The model under review builds one solid part; all positions refer to its coordinate system, in mm. A direction names the side the tool comes from. Round coordinates to 2 decimals unless told otherwise and drop trailing zeros. Write each loop counter-clockwise with the first axis right and the second up, starting at its lowest first coordinate (ties: lowest second). Pieces come first, ordered by that corner, then holes. Notation, with made-up numbers: (27, -36.5) - (34, -36.5) arc R14 cw to (34, -13.5) - close; hole circle Ø6 at (-13.5, 78). An arc over 180 degrees is marked (long way). Return JSON: item names as keys, results as strings.
from build123d import *

# Parameters (mm, degrees)
SALIENTE_EXTRUIR1_DEPTH = 27
CROQUIS3_R              = 4
CROQUIS3_R_2            = 2
SALIENTE_EXTRUIR2_DEPTH = 2
CROQUIS6_R              = 2
CORTAR_EXTRUIR2_DEPTH   = 10
SALIENTE_EXTRUIR4_START = 2
CROQUIS9_R              = 4
CROQUIS9_R_2            = 2
SALIENTE_EXTRUIR4_DEPTH = 2
CORTAR_EXTRUIR3_START   = -10
CROQUIS10_R             = 2
CORTAR_EXTRUIR3_DEPTH   = 10
CROQUIS11_R             = 9.5
SALIENTE_EXTRUIR5_DEPTH = 4.5
SALIENTE_EXTRUIR6_START = 4.5
CROQUIS12_R             = 9.5
SALIENTE_EXTRUIR6_DEPTH = 4.5
CROQUIS13_R             = 4
SALIENTE_EXTRUIR7_DEPTH = 15
CORTAR_EXTRUIR6_START   = -13
CORTAR_EXTRUIR6_DEPTH   = 13
SALIENTE_EXTRUIR8_START = 15
CROQUIS16_R             = 4
SALIENTE_EXTRUIR8_DEPTH = 15
CORTAR_EXTRUIR7_DEPTH   = 13
CROQUIS18_R             = 4
CORTAR_EXTRUIR8_DEPTH   = 20


with BuildPart() as part:
    # Croquis2 → Saliente-Extruir1 (new body)
    with BuildSketch(Plane(origin=(0, 0, 0), x_dir=(1, 0, 0), z_dir=(0, 1, 0))):
        with BuildLine():
            Line((-26.320513929, 20.055), (26.15, 20.055))
            ThreePointArc((26.15, 20.055), (28.26352098, 19.143001272), (29.05, 16.97963275))
            Line((29.05, 16.97963275), (29.05, -16.97963275))
            ThreePointArc((29.05, -16.97963275), (28.26352098, -19.143001272), (26.15, -20.055))
            Line((26.15, -20.055), (-26.320513929, -20.055))
            ThreePointArc((-26.320513929, -20.055), (-28.26710835, -19.146484969), (-29.06, -17.15))
            Line((-29.06, -17.15), (-29.06, 17.15))
            ThreePointArc((-29.06, 17.15), (-28.26710835, 19.146484969), (-26.320513929, 20.055))
        make_face()
    extrude(amount=SALIENTE_EXTRUIR1_DEPTH)

    # Croquis3 → Saliente-Extruir2 (add)
    with BuildSketch(Plane(origin=(0, 27, 0), x_dir=(1, 0, 0), z_dir=(0, 1, 0))):
        with BuildLine():
            Line((22.293849377, -10.723072318), (19.016921695, -8.42922294))
            ThreePointArc((19.016921695, -8.42922294), (13.446144636, -9.412301245), (14.42922294, -14.983078305))
            Line((14.42922294, -14.983078305), (17.706150623, -17.276927682))
            ThreePointArc((17.706150623, -17.276927682), (23.276927682, -16.293849377), (22.293849377, -10.723072318))
        make_face()
        with Locations(Location((-20, 14, 0), (0, 0, 270))):
            Circle(CROQUIS3_R)
        with Locations(Location((20, 14, 0), (0, 0, 270))):
            Circle(CROQUIS3_R)
        with Locations(Location((-20, -14, 0), (0, 0, 270))):
            Circle(CROQUIS3_R)
        with Locations(Location((8, 4, 0), (0, 0, 270))):
            Circle(CROQUIS3_R_2)
        with Locations(Location((8, -4, 0), (0, 0, 270))):
            Circle(CROQUIS3_R_2)
    extrude(amount=SALIENTE_EXTRUIR2_DEPTH)

    # Croquis6 → Cortar-Extruir2 (cut)
    with BuildSketch(Plane(origin=(0, 29, 0), x_dir=(1, 0, 0), z_dir=(0, 1, 0))):
        with Locations(Location((-20, 14, 0), (0, 0, 270))):
            Circle(CROQUIS6_R)
        with Locations(Location((20, 14, 0), (0, 0, 270))):
            Circle(CROQUIS6_R)
        with Locations(Location((20, -14, 0), (0, 0, 270))):
            Circle(CROQUIS6_R)
        with Locations(Location((-20, -14, 0), (0, 0, 270))):
            Circle(CROQUIS6_R)
    extrude(amount=-CORTAR_EXTRUIR2_DEPTH, mode=Mode.SUBTRACT)

    # Croquis9 → Saliente-Extruir4 (add)
    with BuildSketch(Plane.XZ.offset(SALIENTE_EXTRUIR4_START)):
        with Locations(Location((-20, 14, 0), (0, 0, 90))):
            Circle(CROQUIS9_R)
        with Locations(Location((-20, -14, 0), (0, 0, 90))):
            Circle(CROQUIS9_R)
        with Locations(Location((8, 4, 0), (0, 0, 90))):
            Circle(CROQUIS9_R_2)
        with Locations(Location((8, -4, 0), (0, 0, 90))):
            Circle(CROQUIS9_R_2)
        with Locations(Location((20, -14, 0), (0, 0, 90))):
            Circle(CROQUIS9_R)
        with BuildLine():
            Line((14.255148366, 14.861221242), (17.535309468, 17.150444505))
            ThreePointArc((17.535309468, 17.150444505), (23.214821143, 16.380110295), (22.293849377, 10.723072318))
            Line((22.293849377, 10.723072318), (18.838221007, 8.304132458))
            ThreePointArc((18.838221007, 8.304132458), (13.265826422, 9.28952325), (14.255148366, 14.861221242))
        make_face()
    extrude(amount=-SALIENTE_EXTRUIR4_DEPTH)

    # Croquis10 → Cortar-Extruir3 (cut)
    with BuildSketch(Plane.XZ.offset(2).offset(CORTAR_EXTRUIR3_START)):
        with Locations(Location((20, -14, 0), (0, 0, 90))):
            Circle(CROQUIS10_R)
        with Locations(Location((20, 14, 0), (0, 0, 90))):
            Circle(CROQUIS10_R)
        with Locations(Location((-20, 14, 0), (0, 0, 90))):
            Circle(CROQUIS10_R)
        with Locations(Location((-20, -14, 0), (0, 0, 90))):
            Circle(CROQUIS10_R)
    extrude(amount=CORTAR_EXTRUIR3_DEPTH, mode=Mode.SUBTRACT)

    # Croquis11 → Saliente-Extruir5 (add)
    with BuildSketch(Plane(origin=(0, 27, 0), x_dir=(1, 0, 0), z_dir=(0, 1, 0))):
        with Locations(Location((-8.85, 0, 0), (0, 0, 270))):
            Circle(CROQUIS11_R)
    extrude(amount=SALIENTE_EXTRUIR5_DEPTH)

    # Croquis12 → Saliente-Extruir6 (add)
    with BuildSketch(Plane.XZ.offset(SALIENTE_EXTRUIR6_START)):
        with Locations(Location((-8.85, 0, 0), (0, 0, 90))):
            Circle(CROQUIS12_R)
    extrude(amount=-SALIENTE_EXTRUIR6_DEPTH)

    # Croquis13 → Saliente-Extruir7 (add)
    with BuildSketch(Plane(origin=(0, 31.5, 0), x_dir=(1, 0, 0), z_dir=(0, 1, 0))):
        with Locations(Location((-8.85, 0, 0), (0, 0, 270))):
            Circle(CROQUIS13_R)
    extrude(amount=SALIENTE_EXTRUIR7_DEPTH)

    # Croquis15 → Cortar-Extruir6 (cut)
    with BuildSketch(Plane(origin=(0, 46.5, 0), x_dir=(1, 0, 0), z_dir=(0, 1, 0)).offset(CORTAR_EXTRUIR6_START)):
        with BuildLine():
            Line((-5.85, 2.645751311), (-5.85, -2.645751311))
            ThreePointArc((-5.85, -2.645751311), (-4.85, 0), (-5.85, 2.645751311))
        make_face()
    extrude(amount=CORTAR_EXTRUIR6_DEPTH, mode=Mode.SUBTRACT)

    # Croquis16 → Saliente-Extruir8 (add)
    with BuildSketch(Plane.XZ.offset(4.5).offset(SALIENTE_EXTRUIR8_START)):
        with Locations(Location((-8.85, 0, 0), (0, 0, 318.590377891))):
            Circle(CROQUIS16_R)
    extrude(amount=-SALIENTE_EXTRUIR8_DEPTH)

    # Croquis17 → Cortar-Extruir7 (cut)
    with BuildSketch(Plane.XZ.offset(19.5)):
        with BuildLine():
            Line((-5.85, 2.645751311), (-5.85, -2.645751311))
            ThreePointArc((-5.85, -2.645751311), (-4.85, 0), (-5.85, 2.645751311))
        make_face()
    extrude(amount=-CORTAR_EXTRUIR7_DEPTH, mode=Mode.SUBTRACT)

    # Croquis18 → Cortar-Extruir8 (cut)
    with BuildSketch(Plane(origin=(29.05, 0, 0), x_dir=(0, 0, -1), z_dir=(1, 0, 0))):
        with Locations((0, 11.5)):
            Circle(CROQUIS18_R)
    extrude(amount=-CORTAR_EXTRUIR8_DEPTH, mode=Mode.SUBTRACT)


solid = part.part
(1) For faces 5 (the flat face through (8, 29, 4)), 6 (the flat face through (18, -2, 13)), 7 (the cylindrical face through (-22.7, -1.01, -16.95)), 8 (the flat face through (9.05, 12, 0)), 9 (the cylindrical face through (-17.3, 27.99, -16.95)), list the 3-axis set-ups (+Z, -Z, +X, -X, +Y, -Y) from which the entire face can be reached by the end or side of a thin tool; tool diameter is ignored.
Filled in:
{"face 5": "+Z, -Z, +X, +Y", "face 6": "+Z, -Z, +X, -Y", "face 7": "-Y", "face 8": "+X", "face 9": "+Y"}
(2) Add section C-C (y = 11.5). Write out the cut boundary in (x, z) (3 decimals), plus the area to 3 significant figures.
Filled in:
{"outline": "(-29.06, -17.15) arc R2.91 ccw to (-26.321, -20.055) - (26.15, -20.055) arc R2.905 ccw to (29.05, -16.98) - (29.05, -4) - (9.05, -4) - (9.05, 4) - (29.05, 4) - (29.05, 16.98) arc R2.905 ccw to (26.15, 20.055) - (-26.321, 20.055) arc R2.91 ccw to (-29.06, 17.15) - close", "area": "2,160 mm2"}
(3) Mouldability with a two-part tool opening along Y and no side actions: class faces 1 (the cylindrical face through (19.19, 15.466, 0.521)), 2 (the flat face through (8, -2, -4)), 3 (the flat face through (-9, 46.5, 0)), 4 (the flat face through (29.05, 16, 0)) as released by +Y, released by -Y, zero draft, split by the parting line, or undercut.
Filled in:
{"face 1": "undercut", "face 2": "released by -Y", "face 3": "released by +Y", "face 4": "zero draft"}
(4) Add section D-D (z = 5). Write out the cut boundary in (x, y), plus the area to 3 significant figures.
Filled in:
{"outline": "(-29.06, 0) - (-16.93, 0) - (-16.93, -4.5) - (-0.77, -4.5) - (-0.77, 0) - (6.27, 0) - (6.27, -2) - (9.73, -2) - (9.73, 0) - (29.05, 0) - (29.05, 27) - (9.73, 27) - (9.73, 29) - (6.27, 29) - (6.27, 27) - (-0.77, 27) - (-0.77, 31.5) - (-16.93, 31.5) - (-16.93, 27) - (-29.06, 27) - close", "area": "1,730 mm2"}
(5) Add section B-B (z = 0). Write out the cut boundary in (x, y), plus the area to 3 significant figures.
Filled in:
{"outline": "(-29.06, 0) - (-18.35, 0) - (-18.35, -4.5) - (-12.85, -4.5) - (-12.85, -19.5) - (-5.85, -19.5) - (-5.85, -6.5) - (-4.85, -6.5) - (-4.85, -4.5) - (0.65, -4.5) - (0.65, 0) - (29.05, 0) - (29.05, 7.5) - (9.05, 7.5) - (9.05, 15.5) - (29.05, 15.5) - (29.05, 27) - (0.65, 27) - (0.65, 31.5) - (-4.85, 31.5) - (-4.85, 33.5) - (-5.85, 33.5) - (-5.85, 46.5) - (-12.85, 46.5) - (-12.85, 31.5) - (-18.35, 31.5) - (-18.35, 27) - (-29.06, 27) - close", "area": "1,790 mm2"}
(6) Wall thickness on line 1 (Z direction, x = 20, y = 2.5) (3 decimals); line 2 (X direction, y = 20, z = -14); line 3 (Z direction, x = 19.5, y = 4) (1 decimal): over which ranges is each line inside the solid? List them lowest first.
Filled in:
{"line 1": "z = -20.055 to -16, -12 to 12, 16 to 20.055", "line 2": "x = -29.06 to -22, -18 to 18, 22 to 29.05", "line 3": "z = -20.1 to -15.9, -12.1 to 12.1, 15.9 to 20.1"}
(7) Clearance check with flat-ended pins moving along their axes: pin 1 Ø9 at (x, z) = (-19.5, -14) entering from +Y; pin 2 Ø2 at (x, z) = (20, -14.5) entering from -Y; pin 3 Ø1.5 at (x, z) = (-19.5, -8) entering from -Y. State where each tip first meets the part, or that it passes through.
Filled in:
{"pin 1": "stops at y = 29", "pin 2": "stops at y = 8", "pin 3": "stops at y = 0"}
(8) Add section A-A (x = 25). Write out the cut boundary in (y, z) (3 decimals).
Filled in:
{"outline": "(0, -20.055) - (27, -20.055) - (27, 20.055) - (0, 20.055) - close; hole circle Ø8 at (11.5, 0)"}
